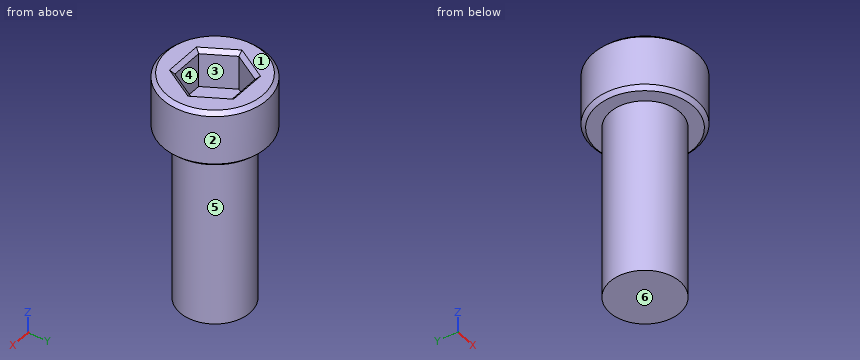
Autodesk Inventor part; units mm, degrees
ref_plane "YZ Plane" through (0, 0, 0) normal (1, 0, 0) x (0, 1, 0)
ref_plane "XZ Plane" through (0, 0, 0) normal (0, 1, 0) x (-1, 0, 0)
ref_plane "XY Plane" through (0, 0, 0) normal (0, 0, 1) x (1, 0, 0)
sketch "Sketch1" plane through (0, 0, 0) normal (0, 0, 1) x (1, 0, 0)
  circle A0 centre (0, 0) radius 3.4925
  circle A1 centre (0, 0) radius 2.3495
  line L0 (2.1997, 0) -> (1.0999, -1.905)
  line L1 (1.0999, -1.905) -> (-1.0999, -1.905)
  line L2 (-1.0999, -1.905) -> (-2.1997, 0)
  line L3 (-2.1997, 0) -> (-1.0999, 1.905)
  line L4 (-1.0999, 1.905) -> (1.0999, 1.905)
  line L5 (1.0999, 1.905) -> (2.1997, 0)
  dimension "d0" = 6.985
  dimension "d1" = 4.699
  dimension "d2" = 3.81
extrude "Extrusion1" add sketch "Sketch1" along normal blind 3.81 contours A0 | A1
extrude "Extrusion2" add sketch "Sketch1" against normal blind 11.811 contours A1 | L0 L1 L2 L3 L4 L5
extrude "Extrusion3" add sketch "Sketch1" along normal blind 1.27 contours L0 L1 L2 L3 L4 L5
thread "Thread1"
chamfer "Chamfer1" distance 0.254 angle 45 8 edges at (-3.4925, 0, 3.81) (-3.4925, 0, 0) (-1.6498, 0.9525, 3.81) (-1.6498, -0.9525, 3.81) (0, -1.905, 3.81) (1.6498, -0.9525, 3.81) (1.6498, 0.9525, 3.81) (0, 1.905, 3.81)
properties part number "Gearbox Hex Machine Screw 4" material "Steel"
For this review, take the finished solid that the model builds, in its own axes (mm). Face numbers are marked on the shaded views. A direction names the side the tool comes from. Give positions to 0.01 mm unless a question says otherwise; leave off trailing zeros. Loops run counter-clockwise (first coordinate to the right, second up) from the corner with the lowest first, then second, coordinate; pieces in that order, holes last. Notation, with made-up numbers: M 4.25,42 L 46.25,42 A16 ccw 46.25,62 Z; hole C 45,72 d8. An arc over 180 degrees is marked long. Answer as a JSON object with one key per item and string values. Group by question number.
Q1. Add section C-C on z = -1.25. Give the boundary of the cut face in (x, y), and give its area (3 significant figures).
Q2. Insertion check: P1, Ø3, axis at y = 1, z = -4, coming from the -X side; P2, Ø1, axis at y = -2, z = -4.5, coming from the +X side; P3, Ø1, axis at x = 1, z = -9.5, coming from the -Y side. Each pin has a flat end and moves straight along its axis. Give the tip position at first contact, or say it passes through.
Q3. For probe 1 along Z at (x, y) = (-3, 0.75); probe 2 along Z at (x, y) = (-1.25, 1.25); probe 3 along Y at (x, z) = (0, -6.5), list the stretches that pass through material, from the lowest coordinate up. Write a range as [from, to].
Q4. Tool access review of the marked faces 4, 5 and 6: name each direction out of +Z, -Z, +X, -X, +Y, -Y from which nothing blocks a thin tool from reaching the whole face with its end or side.
Q5. Mouldability with a two-part tool opening along Y and no side actions: class the marked faces 1, 2 and 3 as +Y half, -Y half, draft (parallel to the pull), parting line (faces both ways), or undercut.
Q6. Add section A-A on z = 2.25. Give the boundary of the cut face in (x, y) (1 decimal), and give its area (3 significant figures).
Checked values:
{
 "1": {"outline": "C 0,0 d4.7", "area": "17.3 mm²"},
 "2": {"P1": "x = -2.35", "P2": "x = 1.81", "P3": "y = -2.3"},
 "3": {"probe 1": "[0, 3.81]", "probe 2": "[-11.81, 1.27]", "probe 3": "[-2.35, 2.35]"},
 "4": {"face 4": "+Z", "face 5": "-Z", "face 6": "-Z, +X, -X, +Y, -Y"},
 "5": {"face 1": "draft", "face 2": "parting line", "face 3": "undercut"},
 "6": {"outline": "C 0,0 d7; hole M -2.2,0 L -1.1,-1.9 L 1.1,-1.9 L 2.2,0 L 1.1,1.9 L -1.1,1.9 Z", "area": "25.7 mm²"}
}
